```python
from build123d import *

# Parameters (mm, degrees)
CROQUIS1_R                 = 3.75
CROQUIS1_W                 = 6
CROQUIS1_H                 = 3.000001037
CROQUIS1_W_2               = 3
SALIENTE_EXTRUIR1_DEPTH    = 3
S_LIDO_MOVER_COPIAR1_ANGLE = 90


with BuildPart() as part:
    # Croquis1 → Saliente-Extruir1 (new body)
    with BuildSketch(Plane.XY):
        Polygon((41630.614837019, 58015.908765172), (41648.614837019, 58015.908765172), (41648.614837019, 58018.908765172), (41663.614837019, 58018.908765172), (41663.614837019, 58015.908765172), (41665.614813532, 58015.908765172), (41665.614813532, 57990.873439675), (41656.89673353, 57990.873439675), (41656.89673353, 57987.873438638), (41665.614813532, 57987.873438638), (41665.614813532, 57970.908765172), (41663.615195237, 57970.908765172), (41663.615195237, 57967.908765172), (41648.615195237, 57967.908765172), (41648.615195237, 57970.908765172), (41631.115195237, 57970.908765172), (41631.115195237, 57967.908765172), (41620.114837019, 57967.908765172), (41620.114837019, 57970.908765172), (41617.614837019, 57970.908765172), (41617.614837019, 57996.908765172), (41614.63346575, 57996.908765172), (41614.63346575, 57999.908765172), (41617.614837019, 57999.908765172), (41617.614837019, 58015.908765172), (41620.114837019, 58015.908765172), (41620.114837019, 58018.908765172), (41624.614837019, 58018.908765172), (41624.614837019, 58015.908765172), (41625.614837019, 58015.908765172), (41625.614837019, 58018.908765172), (41630.614837019, 58018.908765172), align=None)
        with Locations((41642.614837019, 57992.908765172)):
            Circle(CROQUIS1_R, mode=Mode.SUBTRACT)
        with BuildLine():
            Line((41643.614837019, 57982.908765172), (41643.614837019, 57977.908765172))
            ThreePointArc((41643.614837019, 57977.908765172), (41642.614837019, 57976.908765172), (41641.614837019, 57977.908765172))
            Line((41641.614837019, 57977.908765172), (41641.614837019, 57982.908765172))
            ThreePointArc((41641.614837019, 57982.908765172), (41642.614837019, 57983.908765172), (41643.614837019, 57982.908765172))
        make_face(mode=Mode.SUBTRACT)
        with BuildLine():
            Line((41643.614837019, 58007.908765172), (41643.614837019, 58002.908765172))
            ThreePointArc((41643.614837019, 58002.908765172), (41642.614837019, 58001.908765172), (41641.614837019, 58002.908765172))
            Line((41641.614837019, 58002.908765172), (41641.614837019, 58007.908765172))
            ThreePointArc((41641.614837019, 58007.908765172), (41642.614837019, 58008.908765172), (41643.614837019, 58007.908765172))
        make_face(mode=Mode.SUBTRACT)
        with Locations((41626.616584693, 57989.373439157)):
            Rectangle(CROQUIS1_W, CROQUIS1_H, mode=Mode.SUBTRACT)
        with Locations((41621.616584693, 57989.373439157)):
            Rectangle(CROQUIS1_W_2, CROQUIS1_H, mode=Mode.SUBTRACT)
    extrude(amount=SALIENTE_EXTRUIR1_DEPTH)


with BuildPart() as part_1:
    # Sólido-Mover/Copiar1: moved
    add(part.part.rotate(Axis((0, 57992.408765172, 1.5), (-1, 0, 0)), S_LIDO_MOVER_COPIAR1_ANGLE))


solid = part_1.part
```
Model file for the job. Use its own axes, mm. A direction names the side the tool comes from. Give positions to 0.01 mm unless a question says otherwise; leave off trailing zeros. Loops run counter-clockwise (first coordinate to the right, second up) from the corner with the lowest first, then second, coordinate; pieces in that order, holes last. Notation, with made-up numbers: (-31.5, -26.5) - (12.5, -26.5) arc R17 cw to (12.5, -9.5) - close; hole circle Ø8 at (-14, 20.5). An arc over 180 degrees is marked (long way). One line per item, written item: value. Start each with the question number.
1. Pull direction X, two halves, no side cores. Call faces 1 (the flat face through (41648.615, 57992, -23)), 2 (the flat face through (41656.897, 57992, 5)), 3 (the flat face through (41665, 57992, 23)), 4 (the flat face through (41641.615, 57992, 14)): pulls with the +X half, pulls with the -X half, needs draft (parallel to the pull), parting line crosses it, or undercut.
2. Slice it at C-C (z = 1). List the corners of the cut face in (x, y), plus the area to 4 significant figures.
3. Probe L1, parallel to Z at x = 41663.5, y = 57993.65; L2, parallel to X at y = 57993.4, z = -10.5; L3, parallel to Z at x = 41631.5, y = 57991.1. List the from-to ranges inside material, lowest first. Write a range as from..to.
4. Slice it at A-A (z = -12.5). List the corners of the cut face in (x, y), plus the area to 3 significant figures.
5. Slice it at B-B (y = 57992.05). Give the number of separate pieces and of enclosed holes in the cut face, plus the area to 3 significant figures.
6. Pin check, flat tips, straight feed: pin 1 (0.9 mm diameter, centred on y = 57993, z = 4.5, fed in from +X); pin 2 (1.5 mm diameter, centred on y = 57992, z = 5, fed in from -X); pin 3 (10 mm diameter, centred on x = 41642.61, z = 1, fed in from -Y); pin 4 (1.5 mm diameter, centred on y = 57993, z = -23, fed in from +X). Stop position of each tip, or through.
7. Slice it at D-D (x = 41634). List the corners of the cut face in (y, z).
8. Which spindle directions (+Z, -Z, +X, -X, +Y, -Y) get a long thin tool onto all of the face, cutting with end or side? Do faces 5 (the flat face through (41623.117, 57992, 5)), 6 (the flat face through (41648.615, 57992, 25)), 7 (the flat face through (41616, 57992, -3)). Say none if no direction does.
Solution:
1. face 1: undercut
1. face 2: pulls with the +X half
1. face 3: needs draft
1. face 4: undercut
2. outline: (41617.61, 57990.91) - (41638.86, 57990.91) - (41638.86, 57993.91) - (41617.61, 57993.91) - close; (41646.36, 57990.91) - (41665.61, 57990.91) - (41665.61, 57993.91) - (41646.36, 57993.91) - close
2. area: 121.5 mm^2
3. L1: z = -25..3.04, 6.04..26
3. L2: x = 41617.61..41641.61, 41643.61..41665.61
3. L3: z = -22..23
4. outline: (41617.61, 57990.91) - (41641.61, 57990.91) - (41641.61, 57993.91) - (41617.61, 57993.91) - close; (41643.61, 57990.91) - (41665.61, 57990.91) - (41665.61, 57993.91) - (41643.61, 57993.91) - close
4. area: 138 mm^2
5. separate pieces: 1
5. enclosed holes: 5
5. area: 2,200 mm^2
6. pin 1: stops at x = 41656.9
6. pin 2: stops at x = 41617.61
6. pin 3: stops at y = 57990.91
6. pin 4: stops at x = 41663.61
7. outline: (57990.91, -22) - (57993.91, -22) - (57993.91, 23) - (57990.91, 23) - close
8. face 5: +Y, -Y
8. face 6: +Z, +Y, -Y
8. face 7: +Z, -X, +Y, -Y
